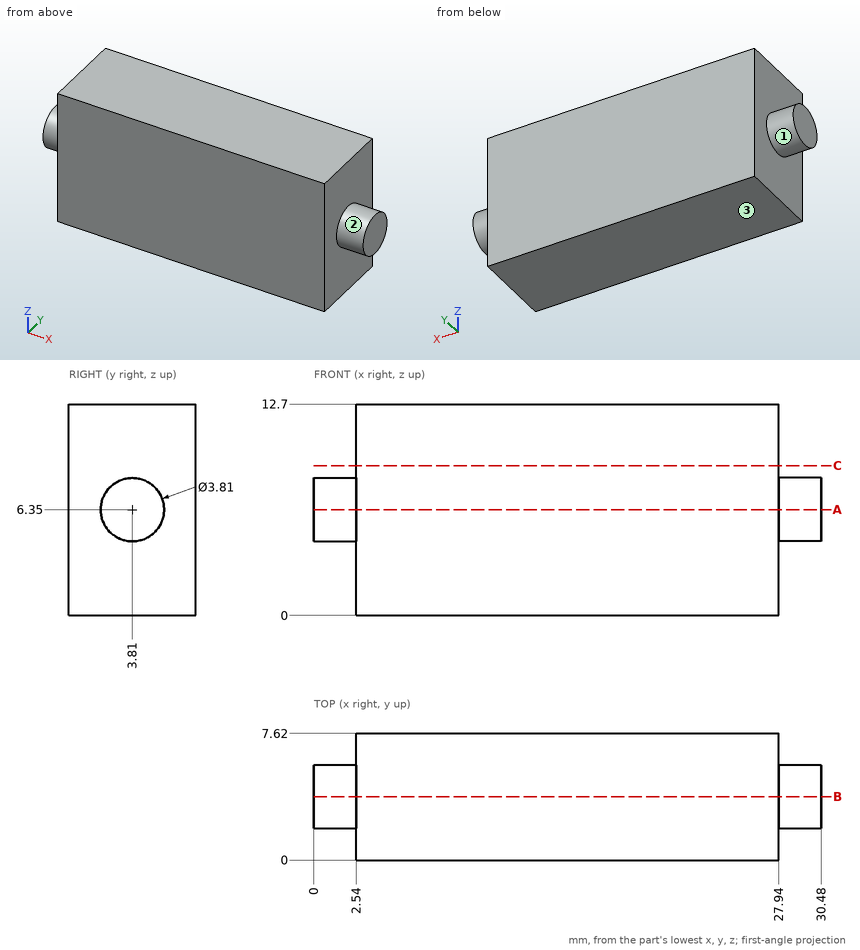
Check sheet for the drawn part. Datum: minimum x, y, z corner. Units: mm. A direction names the side the tool comes from. Coordinates: 2 decimals unless noted, no trailing zeros. Order: outer loops, then holes, each group sorted by start corner. A loop starts at its lowest first (then second) coordinate and runs counter-clockwise, first axis right, second up. Notation, with made-up numbers: M 16.25,19 L 22.25,19 A26 cw 22.25,51 Z; hole C 85.5,-38 d1. An arc over 180 degrees is marked long. One line per item, written item: value. Start each with the question number.
Item 1: Access from +Z, -Z, +X, -X, +Y, -Y to the whole of each face (thin tool, end or side, straight path). Record for the marked faces 1, 2 and 3.
Item 2: Sectioned sample at A-A (z = 6.35). Enter the section's corners in (x, y) (3 decimals).
Item 3: Sectioned sample at B-B (y = 3.81). Enter the section's corners in (x, z) (3 decimals), then the cut area to 3 significant figures.
Item 4: Scan line: probe 1 along X at (y, z) = (2, 4). Record every from-to range of solid material in increasing order.
Item 5: Sectioned sample at C-C (z = 9). Enter the section's corners in (x, y).
Item 6: Gauge pin test, flat end, axial feed: pin 1 (2 mm diameter, centred on y = 6.5, z = 2.5, fed in from -X). Record the tip position at first contact, or that the pin passes through.
Conclusion:
1. face 1: -X
1. face 2: +X
1. face 3: -Z, +X, -X, +Y, -Y
2. outline: M 0,1.905 L 2.54,1.905 L 2.54,0 L 27.94,0 L 27.94,1.905 L 30.48,1.905 L 30.48,5.715 L 27.94,5.715 L 27.94,7.62 L 2.54,7.62 L 2.54,5.715 L 0,5.715 Z
3. outline: M 0,4.445 L 2.54,4.445 L 2.54,0 L 27.94,0 L 27.94,4.445 L 30.48,4.445 L 30.48,8.255 L 27.94,8.255 L 27.94,12.7 L 2.54,12.7 L 2.54,8.255 L 0,8.255 Z
3. area: 342 mm^2
4. probe 1: x = 2.54 to 27.94
5. outline: M 2.54,0 L 27.94,0 L 27.94,7.62 L 2.54,7.62 Z
6. pin 1: stops at x = 2.54
